```python
from build123d import *

# Parameters (mm, degrees)
F2_SIZE  = 2.54
F3_SIZE  = 0.635
F5_DEPTH = 12.7
F7_DEPTH = 12.7


with BuildPart() as f1:
    # F0 (on Front) → F1 (revolve)
    with BuildSketch(Plane.XZ):
        Polygon((4.1783, 10.0584), (4.1783, 0), (10.7442, 0), (10.7442, 46.5836), (10.3632, 46.5836), (10.3632, 48.4886), (10.7442, 48.4886), (10.7442, 62.1284), (7.9629, 62.1284), (7.9629, 10.0584), align=None)
    revolve(axis=Axis((0, 0, 31.0642), (0, 0, 1)))

    # F2
    f2_edges = [f1.edges().sort_by_distance(p)[0] for p in [
        (-10.7442, 0, 0),
    ]]
    chamfer(f2_edges, length=F2_SIZE)

    # F3
    f3_edges = [f1.edges().sort_by_distance(p)[0] for p in [
        (-10.7442, 0, 62.1284),
        (-7.9629, 0, 62.1284),
    ]]
    chamfer(f3_edges, length=F3_SIZE)

    # F4 (on Right) → F5 (cut, symmetric)
    with BuildSketch(Plane.YZ):
        with BuildLine():
            ThreePointArc((0, 13.843), (-1.27, 12.573), (0, 11.303))
            Line((0, 11.303), (0, 12.573))
            Line((0, 12.573), (0, 13.843))
        make_face()
        with BuildLine():
            ThreePointArc((1.27, 23.6982), (-0.8980256121, 24.5962256121), (0, 22.4282))
            ThreePointArc((0, 22.4282), (0.8980256121, 22.8001743879), (1.27, 23.6982))
        make_face()
        with BuildLine():
            Line((0, 12.573), (0, 11.303))
            ThreePointArc((0, 11.303), (0.8980256121, 11.6749743879), (1.27, 12.573))
            ThreePointArc((1.27, 12.573), (0.8980256121, 13.4710256121), (0, 13.843))
            Line((0, 13.843), (0, 12.573))
        make_face()
    extrude(amount=F5_DEPTH, both=True, mode=Mode.SUBTRACT)

    # F6 (on Front) → F7 (cut, symmetric)
    with BuildSketch(Plane.XZ):
        with BuildLine():
            ThreePointArc((0, 11.303), (0.8980256121, 11.6749743879), (1.27, 12.573))
            ThreePointArc((1.27, 12.573), (-0.8980256121, 13.4710256121), (0, 11.303))
        make_face()
    extrude(amount=F7_DEPTH, both=True, mode=Mode.SUBTRACT)


solid = f1.part
```
The listing builds one solid part. Answer for the finished solid, in the listing's coordinates (mm). A direction names the side the tool comes from. Round coordinates to 2 decimals unless told otherwise and drop trailing zeros. Loops run counter-clockwise (first coordinate to the right, second up) from the corner with the lowest first, then second, coordinate; pieces in that order, holes last.
Q1. Section A-A, the plane z = 37 is taken. Determine the outline of the cut face in (x, y).
Q2. Which of the six approach directions +Z, -Z, +X, -X, +Y, -Y give full straight-line access (tool end or side, diameter ignored) to faces 1 (the face through (-2.247, -10.117, 47.549)), 2 (the face through (3.4, -3.4, 10.058)), 3 (the face through (9.925, -4.115, 24.87))?
Q3. Given pin 1 Ø3 at (x, z) = (6, 51.5) entering from -Y; pin 2 Ø8 at (y, z) = (6, 22) entering from +X; pin 3 Ø10 at (y, z) = (6, 23) entering from +X, each flat-ended and moving along its own axis, determine where each tip first touches the part or whether it passes through.
Q4. For a pull along Y with two mould halves and no side action, classify faces 4 (the face through (-2.33, -10.49, 55.08)), 5 (the face through (2.9, 8.3, 62.128)), 6 (the face through (-0.91, -4.08, 4.96)), 7 (the face through (7.356, -3.05, 35.416)) as released by +Y, released by -Y, zero draft, split by the parting line, or undercut.
Q5. Find the intervals of material crossed by line 1 (Y direction, x = 0, z = 47.5); line 2 (Z direction, x = 3, y = 4.25); line 3 (X direction, y = -6.75, z = 54), in increasing order.
Completed:
1. outline: circle Ø21.49 at (0, 0); hole circle Ø15.93 at (0, 0)
2. face 1: none
2. face 2: +Z
2. face 3: +Z, -Z
3. pin 1: stops at y = -9.76
3. pin 2: stops at x = 10.56
3. pin 3: stops at x = 10.7
4. face 4: split by the parting line
4. face 5: zero draft
4. face 6: undercut
4. face 7: undercut
5. line 1: y = -10.36 to -7.96, 7.96 to 10.36
5. line 2: z = 0 to 10.06
5. line 3: x = -8.36 to -4.22, 4.22 to 8.36
